Verification items for the finished model (mm, model axes). Face numbers are marked on the shaded views. A direction names the side the tool comes from. Coordinates: 2 decimals unless noted, no trailing zeros. Order: outer loops, then holes, each group sorted by start corner. A loop starts at its lowest first (then second) coordinate and runs counter-clockwise, first axis right, second up. Notation, with made-up numbers: (2, 40.5) -> (33, 40.5) arc R35 cw to (33, 78.5) -> close; hole circle Ø4 at (76.5, -38.75). An arc over 180 degrees is marked (long way). Use CSV: the item, a comma, the result in double quotes. Start each with the question number.
1) Release check for a two-part mould opening along Y. For the marked faces 1 and 2 record: released by +Y, released by -Y, zero draft, split by the parting line, or undercut.
2) Tool access check on the marked faces 3 and 4. Record the directions out of +Z, -Z, +X, -X, +Y, -Y that give a thin tool (end or side, any length) a straight path to the whole face; none if there is none.
3) Sectioned sample at B-B on x = 168.5. Record the boundary of the cut face in (y, z) (3 decimals), then the cut area to 3 significant figures.
4) Sectioned sample at A-A on z = -15. Record the boundary of the cut face in (x, y), then the cut area to 3 significant figures.
5) Scan lines: line 1 along Z through (x, y) = (20.5, 31) (3 decimals); line 2 along Y through (x, z) = (87.5, -8.5); line 3 along X through (y, z) = (61, -31). Record each from-to range of solid material in increasing order.
6) Sectioned sample at C-C on y = 192.5. Record the boundary of the cut face in (x, z) (3 decimals).
7) Go/stop test with flat-tipped pins: pin 1 (8 mm diameter, centred on x = 6.5, z = -26, fed in from -Y); pin 2 (8 mm diameter, centred on y = 252, z = -18.5, fed in from -X); pin 3 (4 mm diameter, centred on x = 150, y = 150, fed in from +Z); pin 4 (21.5 mm diameter, centred on x = 300, z = -12.5, fed in from +Y). Record where each tip stops, or that it passes through.
from build123d import *

# Parameters (mm, degrees)
SKETCH1_R               = 3.175
BOSS_EXTRUDE1_DEPTH     = 38.1
SKETCH3_W               = 31.75
SKETCH3_H               = 31.75
CUT_EXTRUDE1_DEPTH      = 224.291265993
CUT_EXTRUDE1_DEPTH_BACK = 224.291265993


with BuildPart() as part:
    # Sketch1 → Boss-Extrude1 (new body)
    with BuildSketch(Plane.XY):
        Polygon((19.05, -7.890768363), (307.890768363, 280.95), (280.95, 280.95), (280.95, 307.890768363), (-7.890768363, 19.05), (19.05, 19.05), align=None)
        with Locations((150, 150)):
            Circle(SKETCH1_R, mode=Mode.SUBTRACT)
    extrude(amount=-BOSS_EXTRUDE1_DEPTH)

    # Sketch3 → Cut-Extrude1 (cut, two sides)
    with BuildSketch(Plane(origin=(150, 150, 0), x_dir=(-0.707106781, 0.707106781, 0), z_dir=(-0.707106781, -0.707106781, 0))) as cut_extrude1_sk:
        with Locations((0, 19.05)):
            Rectangle(SKETCH3_W, SKETCH3_H)
    extrude(amount=CUT_EXTRUDE1_DEPTH, mode=Mode.SUBTRACT)
    extrude(cut_extrude1_sk.sketch, amount=-CUT_EXTRUDE1_DEPTH_BACK, mode=Mode.SUBTRACT)


solid = part.part
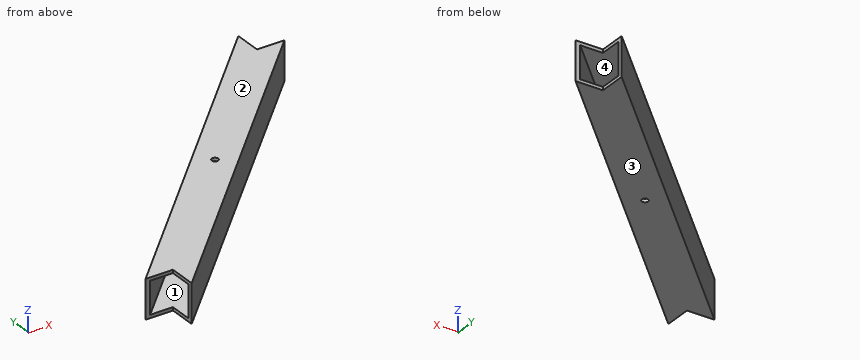
Answers follow:
1,face 1,"undercut"
1,face 2,"zero draft"
2,face 3,"-Z, +X, -X, +Y, -Y"
2,face 4,"none"
3,outline,"(141.559, -38.1) -> (195.441, -38.1) -> (195.441, 0) -> (141.559, 0) -> close; hole (146.049, -34.925) -> (190.951, -34.925) -> (190.951, -3.175) -> (146.049, -3.175) -> close"
3,area,"627 mm²"
4,outline,"(-7.89, 19.05) -> (-3.4, 19.05) -> (280.95, 303.4) -> (280.95, 307.89) -> close; (19.05, -7.89) -> (307.89, 280.95) -> (303.4, 280.95) -> (19.05, -3.4) -> close"
4,area,"2,570 mm²"
5,line 1,"z = -38.1 to -34.925, -3.175 to 0"
5,line 2,"y = 60.56 to 65.05, 109.95 to 114.44"
5,line 3,"x = 34.06 to 38.55, 83.45 to 87.94"
6,outline,"(165.559, -38.1) -> (219.441, -38.1) -> (219.441, 0) -> (165.559, 0) -> close; hole (170.049, -34.925) -> (214.951, -34.925) -> (214.951, -3.175) -> (170.049, -3.175) -> close"
7,pin 1,"stops at y = 24.95"
7,pin 2,"stops at x = 221.06"
7,pin 3,"passes through"
7,pin 4,"stops at y = 280.95"
